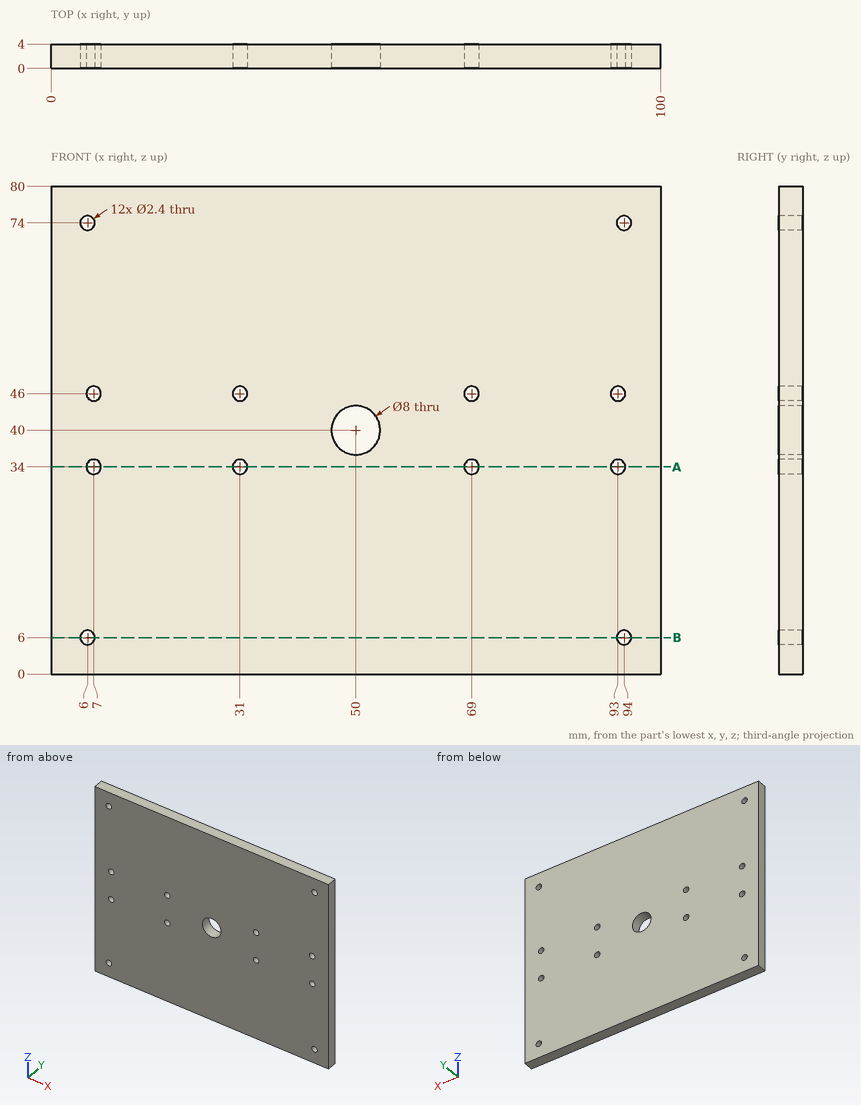
Part print with two shaded views. Sizes in mm from the minimum x, y, z corner. Coordinates: 2 decimals unless noted, no trailing zeros. Order: outer loops, then holes, each group sorted by start corner. A loop starts at its lowest first (then second) coordinate and runs counter-clockwise, first axis right, second up. Notation, with made-up numbers: M 68.5,74.25 L 91.5,74.25 A23 ccw 91.5,108.25 Z; hole C -36.75,40 d5. An arc over 180 degrees is marked long. One line per question, with ' | ' between items. Start each with the question number.
1. Wall check: line 1 along Z through (x, y) = (31, 2.35); line 2 along X through (y, z) = (1, 6); line 3 along Z through (x, y) = (7, 1.05). Give the ranges that are in metal, low to high. Write a range as [from, to].
2. Flat gauge pins, fed straight in: P1, Ø3, axis at x = 31, z = 46, coming from the +Y side; P2, Ø2, axis at x = 94, z = 6, coming from the -Y side. Where does each tip first touch, or does it go through?
3. Cut at A-A (z = 34). Write the cut outline in (x, y).
4. Cut at B-B (z = 6). Write the cut outline in (x, y).
The answers:
1) line 1: z = [0, 32.8], [35.2, 44.8], [47.2, 80] | line 2: x = [0, 4.8], [7.2, 92.8], [95.2, 100] | line 3: z = [0, 5.34], [6.66, 32.8], [35.2, 44.8], [47.2, 73.34], [74.66, 80]
2) P1: stops at y = 4 | P2: passes through
3) outline: M 0,0 L 5.8,0 L 5.8,4 L 0,4 Z; M 8.2,0 L 29.8,0 L 29.8,4 L 8.2,4 Z; M 32.2,0 L 67.8,0 L 67.8,4 L 32.2,4 Z; M 70.2,0 L 91.8,0 L 91.8,4 L 70.2,4 Z; M 94.2,0 L 100,0 L 100,4 L 94.2,4 Z
4) outline: M 0,0 L 4.8,0 L 4.8,4 L 0,4 Z; M 7.2,0 L 92.8,0 L 92.8,4 L 7.2,4 Z; M 95.2,0 L 100,0 L 100,4 L 95.2,4 Z
